CAD build for the part. Positions are in the model's coordinates, mm. A direction names the side the tool comes from. Give positions to 0.01 mm unless a question says otherwise; leave off trailing zeros. Loops run counter-clockwise (first coordinate to the right, second up) from the corner with the lowest first, then second, coordinate; pieces in that order, holes last.
```python
from build123d import *

# Parameters (mm, degrees)
SKETCH1_W           = 170
SKETCH1_H           = 90
BOSS_EXTRUDE1_DEPTH = 5
SKETCH2_R           = 3
BOSS_EXTRUDE2_DEPTH = 50
SKETCH3_R           = 1.55
CUT_EXTRUDE1_DEPTH  = 50


with BuildPart() as part:
    # Sketch1 → Boss-Extrude1 (new body)
    with BuildSketch(Plane(origin=(0, 0, 0), x_dir=(1, 0, 0), z_dir=(0, 1, 0))):
        with Locations((85, 45)):
            Rectangle(SKETCH1_W, SKETCH1_H)
    extrude(amount=BOSS_EXTRUDE1_DEPTH)

    # Sketch2 → Boss-Extrude2 (add)
    with BuildSketch(Plane(origin=(0, 5, 0), x_dir=(1, 0, 0), z_dir=(0, 1, 0))):
        with Locations(Location((5, 85, 0), (0, 0, 90))):
            Circle(SKETCH2_R)
        with Locations(Location((5, 5, 0), (0, 0, 90))):
            Circle(SKETCH2_R)
        with Locations(Location((165, 5, 0), (0, 0, 90))):
            Circle(SKETCH2_R)
        with Locations(Location((165, 85, 0), (0, 0, 90))):
            Circle(SKETCH2_R)
        with Locations(Location((95, 85, 0), (0, 0, 90))):
            Circle(SKETCH2_R)
        with Locations(Location((95, 5, 0), (0, 0, 90))):
            Circle(SKETCH2_R)
    extrude(amount=BOSS_EXTRUDE2_DEPTH)

    # Sketch3 → Cut-Extrude1 (cut)
    with BuildSketch(Plane.XZ):
        with Locations(Location((6.75, -26.75, 0), (0, 0, 270))):
            Circle(SKETCH3_R)
        with Locations(Location((78.25, -26.75, 0), (0, 0, 270))):
            Circle(SKETCH3_R)
        with Locations(Location((78.25, -63.25, 0), (0, 0, 270))):
            Circle(SKETCH3_R)
        with Locations(Location((6.75, -63.25, 0), (0, 0, 270))):
            Circle(SKETCH3_R)
        with Locations(Location((163.25, -63.25, 0), (0, 0, 270))):
            Circle(SKETCH3_R)
        with Locations(Location((91.75, -63.25, 0), (0, 0, 270))):
            Circle(SKETCH3_R)
        with Locations(Location((91.75, -26.75, 0), (0, 0, 270))):
            Circle(SKETCH3_R)
        with Locations(Location((163.25, -26.75, 0), (0, 0, 270))):
            Circle(SKETCH3_R)
    extrude(amount=-CUT_EXTRUDE1_DEPTH, mode=Mode.SUBTRACT)


solid = part.part
```
1. Probe line 1 along X through (y, z) = (2.15, -26.75); line 2 along Z through (x, y) = (78.25, 1.2); line 3 along Z through (x, y) = (91, 2). List the from-to ranges inside material, lowest first.
Responses:
line 1: x = 0 to 5.2, 8.3 to 76.7, 79.8 to 90.2, 93.3 to 161.7, 164.8 to 170
line 2: z = -90 to -64.8, -61.7 to -28.3, -25.2 to 0
line 3: z = -90 to -64.61, -61.89 to -28.11, -25.39 to 0
2. Saw through at B-B, the plane z = -36. List the corners of the cut face in (x, y), and give its area (3 significant figures).
Responses:
outline: (0, 0) - (170, 0) - (170, 5) - (0, 5) - close
area: 850 mm2
3. Saw through at A-A, the plane y = 7.5. List the corners of the cut face in (x, z).
Responses:
outline: circle Ø6 at (5, -85); circle Ø6 at (5, -5); circle Ø6 at (95, -85); circle Ø6 at (95, -5); circle Ø6 at (165, -85); circle Ø6 at (165, -5)
4. Tool access for faces 1 (the face through (7.216, 2.465, -64.728)), 2 (the face through (5, 30, -82)): list every direction of +Z, -Z, +X, -X, +Y, -Y with a clear straight run to the whole face (end or side of a thin tool).
Responses:
face 1: +Y, -Y
face 2: +Y
5. Saw through at C-C, the plane x = 156.5. List the corners of the cut face in (y, z), and give its area (3 significant figures).
Responses:
outline: (0, -90) - (5, -90) - (5, 0) - (0, 0) - close
area: 450 mm2
6. Drop a flat-ended pin along its axis: pin 1 (5 mm diameter, centred on x = 31, z = -24.5, fed in from +Y). Give the stop position or say it passes through.
Responses:
pin 1: stops at y = 5
7. Pull direction Z, two halves, no side cores. Call faces 3 (the face through (84, 2, -90)), 4 (the face through (79.787, 2.465, -26.548)), 5 (the face through (84, 2, 0)), 6 (the face through (170, 2, -44)): released by +Z, released by -Z, zero draft, split by the parting line, or undercut.
Responses:
face 3: released by -Z
face 4: undercut
face 5: released by +Z
face 6: zero draft
